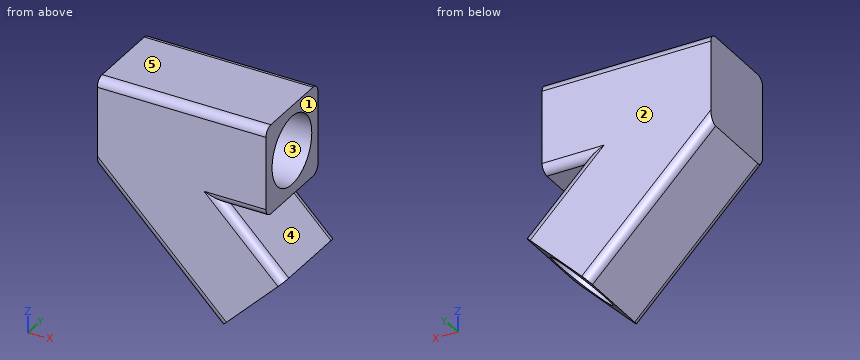
```python
from build123d import *

# Parameters (mm, degrees)
F1_DEPTH = 21.3
F3_R     = 8.15
F4_DEPTH = 35
F2_R     = 8.15
F5_DEPTH = 35
F6_R     = 2


with BuildPart() as f1:
    # F0 (on Front) → F1 (new body)
    with BuildSketch(Plane.XZ):
        Polygon((40, -21.3), (40, -18.8), (24.0872149726, -18.8), (42.4971175493, -37.2099025767), (44.2648845023, -35.4421356237), (30.1227488785, -21.3), align=None)
        Polygon((40, -18.8), (40, -2.5), (2.5, -2.5), (2.5, -20.2644660941), (30.971277016, -48.73574311), (42.4971175493, -37.2099025767), (24.0872149726, -18.8), align=None)
        Polygon((40, 0), (0, 0), (0, -21.3), (29.203510063, -50.503510063), (30.971277016, -48.73574311), (2.5, -20.2644660941), (2.5, -2.5), (40, -2.5), align=None)
    extrude(amount=F1_DEPTH)

    # F3 (on face) → F4 (cut)
    with BuildSketch(Plane(origin=(39.853510063, 0, -39.853510063), x_dir=(0.7071067812, 0, 0.7071067812), z_dir=(0.7071067812, 0, -0.7071067812))):
        with Locations((-4.4113744393, 10.65)):
            Circle(F3_R)
    extrude(amount=-F4_DEPTH, mode=Mode.SUBTRACT)

    # F2 (on face) → F5 (cut)
    with BuildSketch(Plane.YZ.offset(40)):
        with Locations((-10.65, -10.65)):
            Circle(F2_R)
    extrude(amount=-F5_DEPTH, mode=Mode.SUBTRACT)

    # F6
    f6_edges = [f1.edges().sort_by_distance(p)[0] for p in [
        (20, 0, 0),
        (20, -21.3, 0),
        (14.601755, -21.3, -35.901755),
        (14.601755, 0, -35.901755),
        (37.193817, -21.3, -28.371068),
        (37.193817, 0, -28.371068),
        (35.061374, 0, -21.3),
        (35.061374, -21.3, -21.3),
    ]]
    fillet(f6_edges, radius=F6_R)


solid = f1.part
```
Geometry check sheet. Reference: the model listing, model coordinates, mm. Face numbers are marked on the shaded views. A direction names the side the tool comes from. Round coordinates to 2 decimals unless told otherwise and drop trailing zeros. Order: outer loops, then holes, each group sorted by start corner. A loop starts at its lowest first (then second) coordinate and runs counter-clockwise, first axis right, second up. Notation, with made-up numbers: (25, 13) - (32, 13) arc R19 cw to (32, 28) - close; hole circle Ø2 at (-28, 80.5). An arc over 180 degrees is marked (long way). Use a Markdown table: item, result. Add a question column.
(1) Release check for a two-part mould opening along Y. For the marked faces 1, 2 and 3 record: pulls with the +Y half, pulls with the -Y half, needs draft (parallel to the pull), parting line crosses it, or undercut.
(2) Material ranges on line 1 along Z through (x, y) = (27.5, -10.65); line 2 along Z through (x, y) = (12.5, -6); line 3 along X through (y, z) = (-20.5, -4), recorded low to high. Write a range as [from, to].
(3) Sectioned sample at C-C, the plane x = 32. Count the separate pieces of the cut face and the enclosed holes in it, and give its area (3 significant figures).
(4) Sectioned sample at A-A, the plane z = -10.65. Enter the section's corners in (x, y), and give its area (4 significant figures).
(5) Tool access check on the marked faces 4 and 5. Record the directions out of +Z, -Z, +X, -X, +Y, -Y that give a thin tool (end or side, any length) a straight path to the whole face; none if there is none.
(6) Depth check by flat-ended pin: pin 1 (5 mm diameter, centred on y = -8.5, z = -14.5, fed in from +X); pin 2 (10.5 mm diameter, centred on y = -13.5, z = -7.5, fed in from +X); pin 3 (5 mm diameter, centred on y = -10, z = -31, fed in from -X). Enter the tip coordinate at first touch or a pass-through.
(7) Sectioned sample at B-B, the plane y = -10.65. Enter the section's corners in (x, z), and give its area (3 significant figures).
Answers below:
| question | item | result |
|---|---|---|
| 1 | face 1 | needs draft |
| 1 | face 2 | pulls with the +Y half |
| 1 | face 3 | undercut |
| 2 | line 1 | [-48.8, -45.26], [-22.21, -18.8], [-2.5, 0] |
| 2 | line 2 | [-33.8, -28.2], [-17.71, -17.34], [-3.96, 0] |
| 2 | line 3 | [0, 40] |
| 3 | separate pieces | 2 |
| 3 | enclosed holes | 1 |
| 3 | area | 480 mm² |
| 4 | outline | (0, -21.3) - (40, -21.3) - (40, -18.8) - (5, -18.8) - (5, -2.5) - (40, -2.5) - (40, 0) - (0, 0) - close |
| 4 | area | 281.5 mm² |
| 5 | face 4 | +X, +Y, -Y |
| 5 | face 5 | +Z, +X, -X, +Y, -Y |
| 6 | pin 1 | x = 5 |
| 6 | pin 2 | x = 40 |
| 6 | pin 3 | x = 7.2 |
| 7 | outline | (0, -21.3) - (29.2, -50.5) - (30.97, -48.74) - (6.22, -23.99) - (11.41, -18.8) - (5, -18.8) - (5, -2.5) - (40, -2.5) - (40, 0) - (0, 0) - close; (24.09, -18.8) - (42.5, -37.21) - (44.26, -35.44) - (30.12, -21.3) - (40, -21.3) - (40, -18.8) - close |
| 7 | area | 404 mm² |
